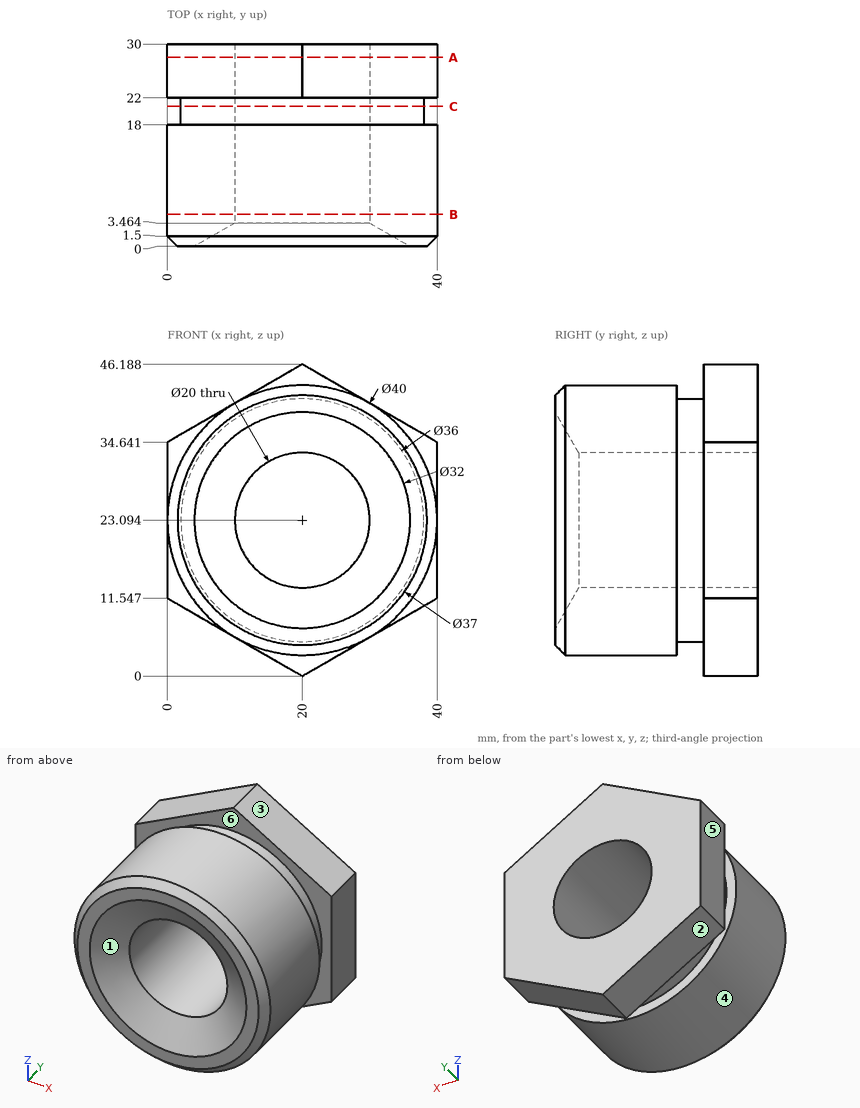
For this review, use the dimensioned drawing (mm, ordinates from the lowest corner) and the shaded views. A direction names the side the tool comes from. Round coordinates to 2 decimals unless told otherwise and drop trailing zeros. Order: outer loops, then holes, each group sorted by start corner. A loop starts at its lowest first (then second) coordinate and runs counter-clockwise, first axis right, second up. Notation, with made-up numbers: M 50,-13 L 58,-13 A16 ccw 58,10 Z; hole C 34,61.25 d10. An arc over 180 degrees is marked long. Use a Markdown table: item, result. Add a question column.
Item 1: Tool access review of the marked faces 4, 5 and 6: name each direction out of +Z, -Z, +X, -X, +Y, -Y from which nothing blocks a thin tool from reaching the whole face with its end or side.
Item 2: Add section B-B, the plane y = 4.75. Give the boundary of the cut face in (x, z).
Item 3: Add section A-A, the plane y = 28. Give the boundary of the cut face in (x, z), then the cut area to 3 significant figures.
Item 4: Mouldability with a two-part tool opening along X and no side actions: class the marked faces 1, 2 and 3 as released by +X, released by -X, zero draft, split by the parting line, or undercut.
Item 5: Add section C-C, the plane y = 20.75. Give the boundary of the cut face in (x, z), then the cut area to 3 significant figures.
Item 6: Insertion check: pin 1 (2 mm diameter, centred on x = 23, z = 9, fed in from -Y); pin 2 (4 mm diameter, centred on y = 13, z = 6, fed in from -X); pin 3 (3 mm diameter, centred on x = 35, y = 25.5, fed in from +Z). Each pin has a flat end and moves straight along its axis. Give the tip position at first contact, or say it passes through.
Item 7: To check wall thickness, follow line 1 along Z through (x, y) = (20, 13.25); line 2 along Z through (x, y) = (20, 19.5); line 3 along X through (y, z) = (23, 23.5). State the ranges of each line that lie inside material, in increasing order.
Geometry results:
| question | item | result |
|---|---|---|
| 1 | face 4 | -Y |
| 1 | face 5 | +Z, -Z, -X, +Y, -Y |
| 1 | face 6 | none |
| 2 | outline | C 20,23.09 d40; hole C 20,23.09 d20 |
| 3 | outline | M 0,11.55 L 20,0 L 40,11.55 L 40,34.64 L 20,46.19 L 0,34.64 Z; hole C 20,23.09 d20 |
| 3 | area | 1,070 mm² |
| 4 | face 1 | undercut |
| 4 | face 2 | released by -X |
| 4 | face 3 | released by +X |
| 5 | outline | C 20,23.09 d36; hole C 20,23.09 d20 |
| 5 | area | 704 mm² |
| 6 | pin 1 | stops at y = 0.34 |
| 6 | pin 2 | stops at x = 6.88 |
| 6 | pin 3 | stops at z = 38.39 |
| 7 | line 1 | z = 3.09 to 13.09, 33.09 to 43.09 |
| 7 | line 2 | z = 5.09 to 13.09, 33.09 to 41.09 |
| 7 | line 3 | x = 0 to 10.01, 29.99 to 40 |
